Design review of the part built by this model. Coordinates are the model's own, in mm. A direction names the side the tool comes from. Coordinates: 2 decimals unless noted, no trailing zeros. Loops run counter-clockwise (first coordinate to the right, second up) from the corner with the lowest first, then second, coordinate; pieces in that order, holes last. Notation, with made-up numbers: (-31.5, 40) - (-10.5, 40) arc R31 ccw to (-10.5, 65) - close; hole circle Ø6 at (17, 84). An arc over 180 degrees is marked (long way). Answer in a Markdown table with one row per item. Add a question column.
(1) To check wall thickness, follow L1, parallel to X at y = 4.5, z = -6; L2, parallel to Y at x = -14, z = -2; L3, parallel to X at y = 0.7, z = -5. State the ranges of each line that lie inside material, in increasing order. Write a range as [from, to].
(2) The part is to be moulded in two halves that separate along Z. For faces 1 (the face through (-16, 0, -5)), 2 (the face through (-13, 1, -10)), 3 (the face through (-30, 1, -2)), 4 (the face through (-15.664, 0.76, -5.325)), say which applies: released by +Z, released by -Z, zero draft, split by the parting line, or undercut.
(3) Clearance check with flat-ended pins moving along their axes: pin 1 (2 mm diameter, centred on x = -20.5, y = 4.5, fed in from -Z); pin 2 (1.1 mm diameter, centred on y = 3.5, z = -3.5, fed in from -X); pin 3 (3 mm diameter, centred on x = -8.5, z = -6, fed in from +Y). State where each tip first meets the part, or that it passes through.
(4) For faces 5 (the face through (-25, 3, -7.75)), 6 (the face through (-25, 7.5, -5)), 7 (the face through (-25, 3, -2.25)), 8 (the face through (-30, 3, -5)), 9 (the face through (-20, 3, -5)), list the 3-axis set-ups (+Z, -Z, +X, -X, +Y, -Y) from which the entire face can be reached by the end or side of a thin tool; tool diameter is ignored.
(5) We need section D-D, the plane y = 3.25. Write out the cut boundary in (x, z), plus the area to 3 significant figures.
(6) We need section A-A, the plane x = -14.2. Write out the cut boundary in (y, z).
(7) We need section C-C, the plane x = -23. Write out the cut boundary in (y, z).
from build123d import *

# Parameters (mm, degrees)
SKETCH1_W           = 31
SKETCH1_H           = 10
BOSS_EXTRUDE1_DEPTH = 1.5
CUT_EXTRUDE1_REACH  = 34.608
SKETCH2_R           = 1.5
SKETCH3_W           = 10
SKETCH3_H           = 5.5
BOSS_EXTRUDE2_DEPTH = 6
FILLET3_R           = 2.25
FILLET4_R           = 5


with BuildPart() as part:
    # Sketch1 → Boss-Extrude1 (new body)
    with BuildSketch(Plane(origin=(0, 0, 0), x_dir=(1, 0, 0), z_dir=(0, 1, 0))):
        with Locations((-15.5, 5)):
            Rectangle(SKETCH1_W, SKETCH1_H)
    extrude(amount=BOSS_EXTRUDE1_DEPTH)

    # Sketch2 → Cut-Extrude1 (cut, up to next)
    with BuildSketch(Plane(origin=(0, 1.5, 0), x_dir=(1, 0, 0), z_dir=(0, 1, 0)), mode=Mode.PRIVATE) as cut_extrude1_sk1:
        with Locations(Location((-14.2, 5, 0), (0, 0, 270))):
            Circle(SKETCH2_R)
    cut_extrude1_tool1 = extrude(cut_extrude1_sk1.sketch, amount=-CUT_EXTRUDE1_REACH, mode=Mode.PRIVATE) & part.part
    add(cut_extrude1_tool1.solids().sort_by_distance((-14.2, 1.5, -5))[0], mode=Mode.SUBTRACT)

    # Sketch3 → Boss-Extrude2 (add)
    with BuildSketch(Plane(origin=(0, 1.5, 0), x_dir=(1, 0, 0), z_dir=(0, 1, 0))):
        with Locations((-25, 5)):
            Rectangle(SKETCH3_W, SKETCH3_H)
    extrude(amount=BOSS_EXTRUDE2_DEPTH)

    # Fillet3
    fillet3_edges = [part.edges().sort_by_distance(p)[0] for p in [
        (-30, 7.5, -5),
        (-25, 7.5, -2.25),
        (-20, 7.5, -5),
        (-25, 7.5, -7.75),
    ]]
    fillet(fillet3_edges, radius=FILLET3_R)

    # Fillet4
    fillet4_edges = [part.edges().sort_by_distance(p)[0] for p in [
        (-31, 0.75, 0),
        (-31, 0.75, -10),
    ]]
    fillet(fillet4_edges, radius=FILLET4_R - 0.0001)  # a hair under: the kernel refuses the full size


solid = part.part
Responses:
| question | item | result |
|---|---|---|
| 1 | L1 | x = [-30, -20] |
| 1 | L2 | y = [0, 1.5] |
| 1 | L3 | x = [-31, -15.7], [-12.7, 0] |
| 2 | face 1 | zero draft |
| 2 | face 2 | released by -Z |
| 2 | face 3 | released by +Z |
| 2 | face 4 | undercut |
| 3 | pin 1 | stops at z = -7.75 |
| 3 | pin 2 | stops at x = -30 |
| 3 | pin 3 | stops at y = 1.5 |
| 4 | face 5 | -Z, +X, -X, +Y |
| 4 | face 6 | +Z, -Z, +X, -X, +Y |
| 4 | face 7 | +Z, +X, -X, +Y |
| 4 | face 8 | +Z, -Z, -X, +Y |
| 4 | face 9 | +Z, -Z, +X, +Y |
| 5 | outline | (-30, -7.75) - (-20, -7.75) - (-20, -2.25) - (-30, -2.25) - close |
| 5 | area | 55.0 mm2 |
| 6 | outline | (0, -10) - (1.5, -10) - (1.5, -6.5) - (0, -6.5) - close; (0, -3.5) - (1.5, -3.5) - (1.5, 0) - (0, 0) - close |
| 7 | outline | (0, -10) - (1.5, -10) - (1.5, -7.75) - (5.25, -7.75) arc R2.25 ccw to (7.5, -5.5) - (7.5, -4.5) arc R2.25 ccw to (5.25, -2.25) - (1.5, -2.25) - (1.5, 0) - (0, 0) - close |
